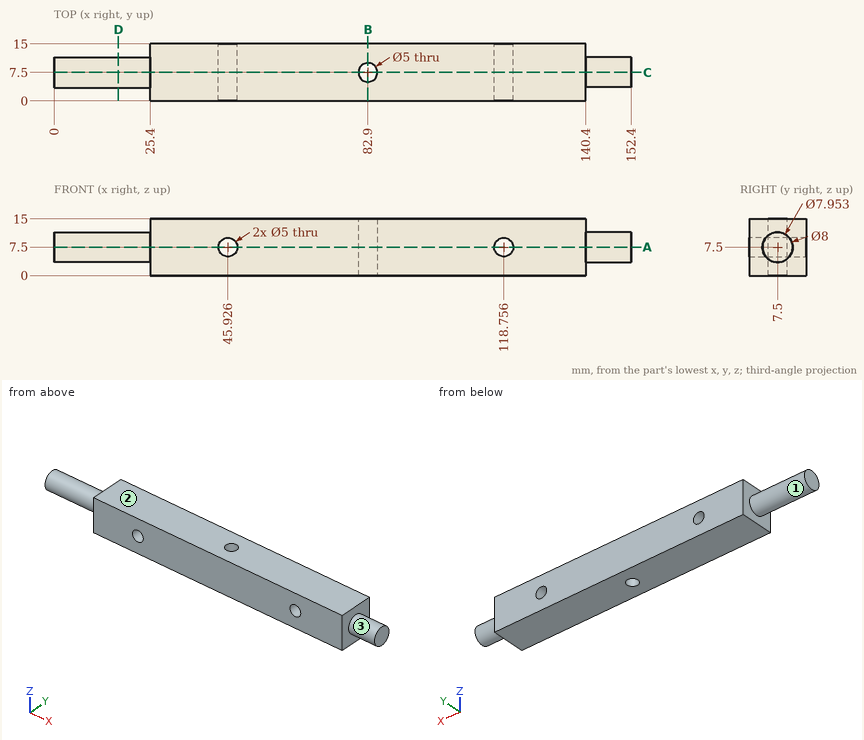
Job drawing, mm, ordinate dimensions from the low corner. One solid piece. A direction names the side the tool comes from. Give positions to 0.01 mm unless a question says otherwise; leave off trailing zeros. Loops run counter-clockwise (first coordinate to the right, second up) from the corner with the lowest first, then second, coordinate; pieces in that order, holes last. Notation, with made-up numbers: (32.25, 24.25) -> (43.25, 24.25) arc R17 ccw to (43.25, 56.25) -> close; hole circle Ø3 at (69.5, 58). An arc over 180 degrees is marked (long way). Use a Markdown table: item, result. Add a question column.
(1) Tool access for the marked faces 1, 2 and 3: list every direction of +Z, -Z, +X, -X, +Y, -Y with a clear straight run to the whole face (end or side of a thin tool).
(2) Slice it at B-B on x = 82.9. List the corners of the cut face in (y, z), and give its area (3 significant figures).
(3) Wall check: line 1 along Y through (x, z) = (83, 11.75); line 2 along X through (y, z) = (10.75, 6) (1 decimal); line 3 along X through (y, z) = (6.5, 8.5) (1 decimal). Give the ranges that are in metal, low to high.
(4) Slice it at A-A on z = 7.5. List the corners of the cut face in (x, y) (1 decimal).
(5) Slice it at C-C on y = 7.5. List the corners of the cut face in (x, z) (1 decimal).
(6) Drop flat-ended pins along their axis: pin 1 Ø1.5 at (y, z) = (6.5, 13.5) entering from +X; pin 2 Ø2 at (y, z) = (12, 4.5) entering from -X. Give the stop position or say it passes through.
(7) Slice it at D-D on x = 17. List the corners of the cut face in (y, z).
Filled sheet:
| question | item | result |
|---|---|---|
| 1 | face 1 | -X |
| 1 | face 2 | +Z, +X, -X, +Y, -Y |
| 1 | face 3 | +X |
| 2 | outline | (0, 0) -> (5, 0) -> (5, 15) -> (0, 15) -> close; (10, 0) -> (15, 0) -> (15, 15) -> (10, 15) -> close |
| 2 | area | 150 mm2 |
| 3 | line 1 | 0 to 5, 10 to 15 |
| 3 | line 2 | 0 to 43.9, 47.9 to 116.8, 120.8 to 152.4 |
| 3 | line 3 | 0 to 43.6, 48.2 to 80.6, 85.2 to 116.5, 121 to 152.4 |
| 4 | outline | (0, 3.5) -> (25.4, 3.5) -> (25.4, 0) -> (43.4, 0) -> (43.4, 15) -> (25.4, 15) -> (25.4, 11.5) -> (0, 11.5) -> close; (48.4, 0) -> (116.3, 0) -> (116.3, 15) -> (48.4, 15) -> close; (121.3, 0) -> (140.4, 0) -> (140.4, 3.5) -> (152.4, 3.5) -> (152.4, 11.5) -> (140.4, 11.5) -> (140.4, 15) -> (121.3, 15) -> close; hole circle Ø5 at (82.9, 7.5) |
| 5 | outline | (0, 3.5) -> (25.4, 3.5) -> (25.4, 0) -> (80.4, 0) -> (80.4, 15) -> (25.4, 15) -> (25.4, 11.5) -> (0, 11.5) -> close; (85.4, 0) -> (140.4, 0) -> (140.4, 3.5) -> (152.4, 3.5) -> (152.4, 11.5) -> (140.4, 11.5) -> (140.4, 15) -> (85.4, 15) -> close; hole circle Ø5 at (45.9, 7.5); hole circle Ø5 at (118.8, 7.5) |
| 6 | pin 1 | x = 140.4 |
| 6 | pin 2 | x = 25.4 |
| 7 | outline | circle Ø8 at (7.5, 7.5) |
